```python
from build123d import *

# Parameters (mm, degrees)
SKETCH2_R           = 6.0325
BOSS_EXTRUDE1_DEPTH = 3.175
SKETCH3_R           = 1.5875
BOSS_EXTRUDE2_DEPTH = 3.175
SKETCH5_W           = 12.065
SKETCH5_H           = 12.065
BOSS_EXTRUDE3_DEPTH = 2.54
BOSS_EXTRUDE4_DEPTH = 6.0325


with BuildPart() as part:
    # Sketch2 → Boss-Extrude1 (new body)
    with BuildSketch(Plane(origin=(0, 0, 0), x_dir=(0, 0, -1), z_dir=(1, 0, 0))):
        Circle(SKETCH2_R)
    extrude(amount=BOSS_EXTRUDE1_DEPTH)

    # Sketch3 → Boss-Extrude2 (add)
    with BuildSketch(Plane(origin=(3.175, 0, 0), x_dir=(0, 0, -1), z_dir=(1, 0, 0))):
        Circle(SKETCH3_R)
    extrude(amount=BOSS_EXTRUDE2_DEPTH)

    # Sketch4 → Revolve1 (revolve)
    with BuildSketch(Plane.XY):
        with BuildLine():
            Line((5.715, 0), (14.351, 0))
            ThreePointArc((14.351, 0), (10.033, 4.318), (5.715, 0))
        make_face()
    revolve(axis=Axis((5.715, 0, 0), (1, 0, 0)))

    # Sketch5 → Boss-Extrude3 (add)
    with BuildSketch(Plane.ZY):
        Rectangle(SKETCH5_W, SKETCH5_H)
    extrude(amount=BOSS_EXTRUDE3_DEPTH)

    # Sketch7 → Boss-Extrude4 (add, symmetric)
    with BuildSketch(Plane.XY):
        with BuildLine():
            Line((-2.54, 6.0325), (-10.935574209, 4.328993713))
            ThreePointArc((-10.935574209, 4.328993713), (-12.148502267, 4.411480747), (-13.149077484, 5.102022434))
            ThreePointArc((-13.149077484, 5.102022434), (-15.862491492, 6.641192846), (-18.922091819, 6.0325))
            ThreePointArc((-18.922091819, 6.0325), (-21.686103075, 5.165714471), (-24.528789325, 5.7226797))
            Line((-24.528789325, 5.7226797), (-27.94, 7.027138907))
            Line((-27.94, 7.027138907), (-28.10330212, 6.600097624))
            Line((-28.10330212, 6.600097624), (-24.708214464, 5.301803917))
            ThreePointArc((-24.708214464, 5.301803917), (-21.651931317, 4.709711596), (-18.682120225, 5.64334004))
            ThreePointArc((-18.682120225, 5.64334004), (-15.935242742, 6.189818173), (-13.499167749, 4.807966919))
            ThreePointArc((-13.499167749, 4.807966919), (-12.299243569, 3.979845601), (-10.844658565, 3.880924315))
            Line((-10.844658565, 3.880924315), (-2.449084356, 5.584430602))
            Line((-2.449084356, 5.584430602), (-2.54, 6.0325))
        make_face()
        with BuildLine():
            Line((-24.528789325, -5.7226797), (-27.94, -7.027138907))
            Line((-27.94, -7.027138907), (-28.10330212, -6.600097624))
            Line((-28.10330212, -6.600097624), (-24.708214464, -5.301803917))
            ThreePointArc((-24.708214464, -5.301803917), (-21.651931317, -4.709711596), (-18.682120225, -5.64334004))
            ThreePointArc((-18.682120225, -5.64334004), (-15.935242742, -6.189818173), (-13.499167749, -4.807966919))
            ThreePointArc((-13.499167749, -4.807966919), (-12.299243569, -3.979845601), (-10.844658565, -3.880924315))
            Line((-10.844658565, -3.880924315), (-2.449084356, -5.584430602))
            Line((-2.449084356, -5.584430602), (-2.54, -6.0325))
            Line((-2.54, -6.0325), (-10.935574209, -4.328993713))
            ThreePointArc((-10.935574209, -4.328993713), (-12.148502267, -4.411480747), (-13.149077484, -5.102022434))
            ThreePointArc((-13.149077484, -5.102022434), (-15.862491492, -6.641192846), (-18.922091819, -6.0325))
            ThreePointArc((-18.922091819, -6.0325), (-21.686103075, -5.165714471), (-24.528789325, -5.7226797))
        make_face()
    extrude(amount=BOSS_EXTRUDE4_DEPTH, both=True)


solid = part.part
```
Work out the finished part from the listing and answer in its coordinate system (mm). A direction names the side the tool comes from. Round coordinates to 2 decimals unless told otherwise and drop trailing zeros. Loops run counter-clockwise (first coordinate to the right, second up) from the corner with the lowest first, then second, coordinate; pieces in that order, holes last. Notation, with made-up numbers: (-24, 70) -> (-20, 70) arc R21 cw to (-20, 76) -> close; hole circle Ø8 at (42.25, -16.5). An arc over 180 degrees is marked (long way). Write each question's results on one line, items separated by ' | '. Start each with the question number.
1. For a pull along Y with two mould halves and no side action, classify faces 5 (the face through (-12.132, -4.406, 0.084)), 6 (the face through (-6.8, -4.7, 0.1)), 7 (the face through (-12.132, 4.406, -0.084)) as +Y half, -Y half, draft (parallel to the pull), parting line (faces both ways), or undercut.
2. A tool of negligible diameter and unlimited length cuts with its end or side. For faces 1 (the face through (-6.679, 5.193, -0.084)), 2 (the face through (-16, 6.2, -0.1)), 3 (the face through (-1, -6.032, 0)), 4 (the face through (0, 5, 5)), from which of +Z, -Z, +X, -X, +Y, -Y can it reach the whole face along a straight path? Write none if from no direction.
3. Find the intervals of material crossed by probe 1 along Y at (x, z) = (-7.5, -1.25); probe 2 along Y at (x, z) = (-15, 3.25); probe 3 along X at (y, z) = (-2, -4.25) (3 decimals), in increasing order. Write a range as from..to.
4. Section A-A (x = -23) is taken. Determine the outline of the cut face in (y, z).
5. Given pin 1 Ø3 at (x, z) = (4, 0.5) entering from +Y; pin 2 Ø3 at (x, z) = (-1, -0.5) entering from -Y; pin 3 Ø5 at (y, z) = (-2, 2.5) entering from +X; pin 4 Ø6 at (x, y) = (-14, -3) entering from +Z, each flat-ended and moving along its own axis, determine where each tip first touches the part or whether it passes through.
6. Section C-C (x = -2) is taken. Determine the outline of the cut face in (y, z).
Evaluation:
1) face 5: -Y half | face 6: undercut | face 7: +Y half
2) face 1: +Z, -Z, +Y | face 2: +Z, -Z | face 3: +Z, -Z, +X, -Y | face 4: +Z, +X, +Y
3) probe 1: y = -5.03..-4.56, 4.56..5.03 | probe 2: y = -6.41..-5.92, 5.92..6.41 | probe 3: x = -2.54..3.175
4) outline: (-5.24, -6.03) -> (-4.78, -6.03) -> (-4.78, 6.03) -> (-5.24, 6.03) -> close; (4.78, -6.03) -> (5.24, -6.03) -> (5.24, 6.03) -> (4.78, 6.03) -> close
5) pin 1: stops at y = 6.03 | pin 2: stops at y = -6.03 | pin 3: stops at x = 14.29 | pin 4: stops at z = 6.03
6) outline: (-6.03, -6.03) -> (6.03, -6.03) -> (6.03, 6.03) -> (-6.03, 6.03) -> close
